Here's how the part is built. I have some questions about the finished solid (model axes, mm). Round coordinates to 2 decimals unless told otherwise and drop trailing zeros. Write each loop counter-clockwise with the first axis right and the second up, starting at its lowest first coordinate (ties: lowest second). Pieces come first, ordered by that corner, then holes. Notation, with made-up numbers: (7.25, 55) -> (22.25, 55) arc R33 ccw to (22.25, 87) -> close; hole circle Ø10 at (71, 82). An arc over 180 degrees is marked (long way). Put each result on its own line as item: value. Start each with the question number.
1) Will these pins go through, and if not, where does the flat tip stop? P1, Ø2, axis at x = 5.5, y = 3, coming from the +Z side; P2, Ø1, axis at x = -5.5, y = 3.5, coming from the +Z side; P3, Ø3, axis at x = -2, y = 4, coming from the +Z side; P4, Ø8, axis at x = 0, z = -60.325, coming from the +Y side.
2) I want a section at A-A, the plane x = 0. List the corners of the cut face in (y, z) for me (3 decimals).
3) If I drill on line 1 along Z through (x, y) = (-0.25, 1); line 2 along Z through (x, y) = (6.75, 3.5); line 3 along Z through (x, y) = (-4, 5.75), over which ranges is the centre line in solid material (lowest first)? Write a range as [from, to].
4) I want a section at B-B, the plane y = 1. List the corners of the cut face in (x, z) for me (3 decimals).
5) We'd pull the mould along Z, two halves only. Please class faces 1 (the cylindrical face through (0.15, 3.13, -63.75)), 2 (the flat face through (0, 6.35, -1)), 3 (the cylindrical face through (6.51, 3.13, -71.02)), 4 (the cylindrical face through (-0.15, 3.13, 63.75)): released by +Z, released by -Z, zero draft, split by the parting line, or undercut.
from build123d import *

# Parameters (mm, degrees)
SKETCH1_R           = 73.025
SKETCH1_R_2         = 3.429
BOSS_EXTRUDE1_DEPTH = 6.35
SKETCH2_W           = 64.77
SKETCH2_H           = 146.05
CUT_EXTRUDE1_DEPTH  = 104.467984179
FILLET1_R           = 6.35


with BuildPart() as part:
    # Sketch1 → Boss-Extrude1 (new body)
    with BuildSketch(Plane(origin=(0, 0, 0), x_dir=(1, 0, 0), z_dir=(0, 1, 0))):
        with Locations(Location((0, 0, 0), (0, 0, 270))):
            Circle(SKETCH1_R)
        with Locations(Location((0, 60.325, 0), (0, 0, 270))):
            Circle(SKETCH1_R_2, mode=Mode.SUBTRACT)
        with Locations(Location((0, -60.325, 0), (0, 0, 90))):
            Circle(SKETCH1_R_2, mode=Mode.SUBTRACT)
    extrude(amount=BOSS_EXTRUDE1_DEPTH)

    # Sketch2 → Cut-Extrude1 (cut, through all)
    with BuildSketch(Plane(origin=(0, 6.35, 0), x_dir=(1, 0, 0), z_dir=(0, 1, 0))):
        with Locations((40.64, 0)):
            Rectangle(SKETCH2_W, SKETCH2_H)
        with Locations((-40.64, 0)):
            Rectangle(SKETCH2_W, SKETCH2_H)
    extrude(amount=-CUT_EXTRUDE1_DEPTH, mode=Mode.SUBTRACT)

    # Fillet1
    fillet1_edges = [part.edges().sort_by_distance(p)[0] for p in [
        (-8.255, 3.175, -72.556912834),
        (-8.255, 3.175, 72.556912834),
        (8.255, 3.175, 72.556912834),
        (8.255, 3.175, -72.556912834),
    ]]
    fillet(fillet1_edges, radius=FILLET1_R)


solid = part.part
Findings:
1. P1: stops at z = 72.44
1. P2: stops at z = 72.19
1. P3: stops at z = 73.02
1. P4: stops at y = 6.35
2. outline: (0, -73.025) -> (6.35, -73.025) -> (6.35, -63.754) -> (0, -63.754) -> close; (0, -56.896) -> (6.35, -56.896) -> (6.35, 56.896) -> (0, 56.896) -> close; (0, 63.754) -> (6.35, 63.754) -> (6.35, 73.025) -> (0, 73.025) -> close
3. line 1: z = [-73.02, -63.74], [-56.91, 56.91], [63.74, 73.02]
3. line 2: z = [-70.75, 70.75]
3. line 3: z = [-72.64, 72.64]
4. outline: (-8.255, -66.648) arc R6.35 ccw to (-2.086, -72.995) arc R73.025 ccw to (2.086, -72.995) arc R6.35 ccw to (8.255, -66.648) -> (8.255, 66.648) arc R6.35 ccw to (2.086, 72.995) arc R73.025 ccw to (-2.086, 72.995) arc R6.35 ccw to (-8.255, 66.648) -> close; hole circle Ø6.858 at (0, -60.325); hole circle Ø6.858 at (0, 60.325)
5. face 1: undercut
5. face 2: zero draft
5. face 3: released by -Z
5. face 4: undercut
